from build123d import *

# Parameters (mm, degrees)
BOSS_EXTRUDE1_DEPTH       = 4.7625
F_8_32_TAPPED_HOLE1_D     = 3.4544
F_8_32_TAPPED_HOLE1_DEPTH = 8.89
F_8_32_TAPPED_HOLE1_TIP   = 1.037806461
BOSS_EXTRUDE2_DEPTH       = 9.525
SKETCH5_W                 = 6.4262
SKETCH5_H                 = 22.225
CUT_EXTRUDE1_DEPTH        = 6.223
CUT_EXTRUDE2_DEPTH        = 1.5875
CUT_EXTRUDE4_DEPTH        = 5.7625
CUT_EXTRUDE4_DEPTH_BACK   = 5.7625
FILLET1_R                 = 1.524
BOSS_EXTRUDE3_DEPTH       = 6.35
FILLET2_R                 = 0.254
CUT_EXTRUDE5_DEPTH        = 8.9375


with BuildPart() as part:
    # Sketch1 → Boss-Extrude1 (new body, symmetric)
    with BuildSketch(Plane(origin=(0, 0, 0), x_dir=(0, 0, -1), z_dir=(1, 0, 0))):
        with BuildLine():
            Line((-18.389854, 0), (18.389854, 0))
            Line((18.389854, 0), (18.389854, -18.35404))
            ThreePointArc((18.389854, -18.35404), (3.13664885, -20.715801882), (-11.682560966, -25.031958383))
            Line((-11.682560966, -25.031958383), (-18.389854, 0))
        make_face()
    extrude(amount=BOSS_EXTRUDE1_DEPTH, both=True)

    # #8-32 Tapped Hole1
    with Locations(Plane(origin=(0, 0, 0), x_dir=(-1, 0, 0), z_dir=(0, 1, 0))):
        with Locations((0, 12.090146)):
            Hole(F_8_32_TAPPED_HOLE1_D / 2, depth=F_8_32_TAPPED_HOLE1_DEPTH)
            with Locations((0, 0, -(F_8_32_TAPPED_HOLE1_DEPTH + F_8_32_TAPPED_HOLE1_TIP / 2))):  # 118° drill point
                Cone(0, F_8_32_TAPPED_HOLE1_D / 2, F_8_32_TAPPED_HOLE1_TIP, mode=Mode.SUBTRACT)

    # Sketch4 → Boss-Extrude2 (add)
    with BuildSketch(Plane(origin=(4.7625, 0, 0), x_dir=(0, 0, -1), z_dir=(1, 0, 0))):
        with BuildLine():
            Line((18.389854, 0), (24.739854, 0))
            Line((24.739854, 0), (24.739854, -17.95993887))
            ThreePointArc((24.739854, -17.95993887), (21.562219751, -18.114544788), (18.389854, -18.35404))
            Line((18.389854, -18.35404), (18.389854, 0))
        make_face()
    extrude(amount=-BOSS_EXTRUDE2_DEPTH)

    # Sketch5 → Cut-Extrude1 (cut)
    with BuildSketch(Plane(origin=(0, 0, -24.739854), x_dir=(-1, 0, 0), z_dir=(0, 0, -1))):
        with Locations((0, -11.1125)):
            Rectangle(SKETCH5_W, SKETCH5_H)
    extrude(amount=-CUT_EXTRUDE1_DEPTH, mode=Mode.SUBTRACT)

    # Sketch6 → Cut-Extrude2 (cut)
    with BuildSketch(Plane(origin=(4.7625, -3.455581552, 12.676714301), x_dir=(0, -0.262996683, 0.964796738), z_dir=(-1, 0, 0))):
        with BuildLine():
            Line((4.603212059, 4.836470596), (-1.739365308, 3.107529419))
            Line((-1.739365308, 3.107529419), (-1.636225637, -20.725696455))
            ThreePointArc((-1.636225637, -20.725696455), (1.5419234, -20.859537189), (4.715359636, -21.078277005))
            Line((4.715359636, -21.078277005), (4.603212059, 4.836470596))
        make_face()
    cut_extrude2 = extrude(amount=CUT_EXTRUDE2_DEPTH, mode=Mode.SUBTRACT)

    # Mirror1: Cut-Extrude2 across plane
    add(cut_extrude2.mirror(Plane(origin=(0, 0, 0), x_dir=(0, 0, 1), z_dir=(1, 0, 0))), mode=Mode.SUBTRACT)

    # Sketch8 → Cut-Extrude4 (cut, two sides)
    with BuildSketch(Plane(origin=(0, 0, 0), x_dir=(0, 0, -1), z_dir=(1, 0, 0))) as cut_extrude4_sk:
        with BuildLine():
            Line((-8.120493812, -1.524), (17.119854, -1.524))
            Line((17.119854, -1.524), (17.119854, -16.942404249))
            ThreePointArc((17.119854, -16.942404249), (6.985210432, -18.377350774), (-2.991129125, -20.667049623))
            Line((-2.991129125, -20.667049623), (-8.120493812, -1.524))
        make_face()
    extrude(amount=CUT_EXTRUDE4_DEPTH, mode=Mode.SUBTRACT)
    extrude(cut_extrude4_sk.sketch, amount=-CUT_EXTRUDE4_DEPTH_BACK, mode=Mode.SUBTRACT)

    # Fillet1
    fillet1_edges = [part.edges().sort_by_distance(p)[0] for p in [
        (0, -20.667049623, 2.991129125),
        (0, -1.524, 8.120493812),
        (0, -1.524, -17.119854),
        (0, -16.942404249, -17.119854),
    ]]
    fillet(fillet1_edges, radius=FILLET1_R)

    # Sketch9 → Boss-Extrude3 (add)
    with BuildSketch(Plane(origin=(3.175, 0, 0), x_dir=(0, 0, -1), z_dir=(1, 0, 0))):
        Polygon((-18.389854, 0), (-21.676855873, 0), (-21.095098292, -2.171148848), (-18.028283794, -1.349398379), align=None)
    extrude(amount=-BOSS_EXTRUDE3_DEPTH)

    # Fillet2
    fillet2_edges = [part.edges().sort_by_distance(p)[0] for p in [
        (0, -2.171148848, 21.095098292),
    ]]
    fillet(fillet2_edges, radius=FILLET2_R)

    # Sketch13 → Cut-Extrude5 (cut, through all)
    with BuildSketch(Plane(origin=(3.175, 0, 0), x_dir=(0, 0, -1), z_dir=(1, 0, 0))):
        with BuildLine():
            Line((-17.905611214, -1.316528361), (-18.028283794, -1.349398379))
            Line((-18.028283794, -1.349398379), (-11.682560966, -25.031958383))
            ThreePointArc((-11.682560966, -25.031958383), (-11.622647023, -25.010220768), (-11.562721445, -24.988515246))
            Line((-11.562721445, -24.988515246), (-17.905611214, -1.316528361))
        make_face()
    extrude(amount=-CUT_EXTRUDE5_DEPTH, mode=Mode.SUBTRACT)


solid = part.part
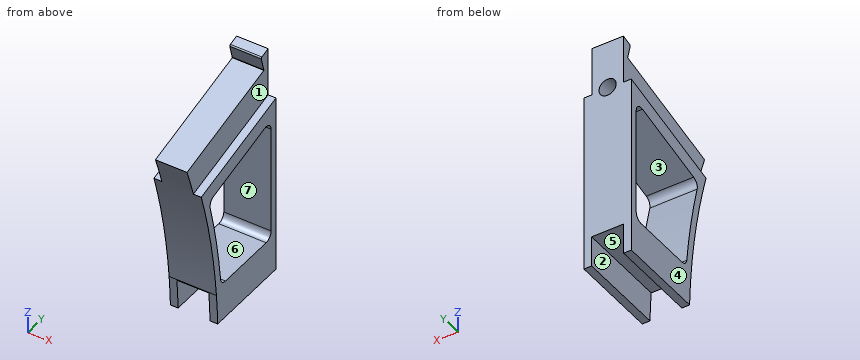
The listing builds one solid part. Answer for the finished solid, in the listing's coordinates (mm). Face numbers are marked on the shaded views. A direction names the side the tool comes from. Coordinates: 2 decimals unless noted, no trailing zeros. Write each loop counter-clockwise with the first axis right and the second up, starting at its lowest first coordinate (ties: lowest second). Pieces come first, ordered by that corner, then holes. Notation, with made-up numbers: (32.25, 27.25) - (57.25, 27.25) arc R14 cw to (57.25, 40.25) - close; hole circle Ø4 at (85, 22.25). An arc over 180 degrees is marked (long way). Put each result on its own line as item: value.
1. The part is cut by section D-D on y = -13.5. Give the vertices of the cut face in (x, z) (1 decimal), plus the area to 3 significant figures.
Answer sheet:
outline: (-4.8, -24.7) - (-3.2, -24.7) - (-3.2, -18.5) - (3.2, -18.5) - (3.2, -24.7) - (4.8, -24.7) - (4.8, -17.1) - (-4.8, -17.1) - close; (-4.8, 4.9) - (4.8, 4.9) - (4.8, 8.2) - (3.2, 8.2) - (3.2, 14.6) - (-3.2, 14.6) - (-3.2, 8.2) - (-4.8, 8.2) - close
area: 105 mm^2
2. The part is cut by section C-C on z = -2.5. Give the vertices of the cut face in (x, y), plus the area to 3 significant figures.
Answer sheet:
outline: (-4.76, -20.86) - (4.76, -20.86) - (4.76, -19.3) - (-4.76, -19.3) - close; (-4.76, -1.52) - (4.76, -1.52) - (4.76, 0) - (-4.76, 0) - close
area: 29.4 mm^2
3. Flat-ended cylindrical pins translate along their axes: pin 1 Ø2 at (x, z) = (0, 12.09) entering from -Y; pin 2 Ø8 at (y, z) = (-14.5, 13) entering from -X (3 decimals); pin 3 Ø5 at (x, y) = (0.5, -6.5) entering from +Z. Find the tip coordinate at first contact, or state that the pin passes through.
Answer sheet:
pin 1: stops at y = -24.99
pin 2: stops at x = -3.175
pin 3: stops at z = 17.19
4. The part is cut by section B-B on x = 4. Give the vertices of the cut face in (y, z) (1 decimal).
Answer sheet:
outline: (-23, 5.6) arc R119 cw to (-18.4, -18.4) arc R119 cw to (-18, -24.7) - (0, -24.7) - (0, 11.8) - close; hole (-20.3, 1.5) arc R120.5 cw to (-17.1, -15.8) arc R1.5 ccw to (-15.6, -17.1) - (-3, -17.1) arc R1.5 ccw to (-1.5, -15.6) - (-1.5, 6.1) arc R1.5 ccw to (-3.4, 7.6) - (-19.2, 3.4) arc R1.5 ccw to start
5. Determine the mould class of the marked faces 4, 5, 6 and 7 for opening direction Z: pulls with the +Z half, pulls with the -Z half, needs draft (parallel to the pull), parting line crosses it, or undercut.
Answer sheet:
face 4: needs draft
face 5: pulls with the -Z half
face 6: undercut
face 7: undercut
6. The part is cut by section A-A on y = -6.25. Give the vertices of the cut face in (x, z) (1 decimal), plus the area to 3 significant figures.
Answer sheet:
outline: (-4.8, -24.7) - (-3.2, -24.7) - (-3.2, -18.5) - (3.2, -18.5) - (3.2, -24.7) - (4.8, -24.7) - (4.8, -17.1) - (-4.8, -17.1) - close; (-4.8, 6.9) - (4.8, 6.9) - (4.8, 10.1) - (3.2, 10.1) - (3.2, 16.6) - (-3.2, 16.6) - (-3.2, 10.1) - (-4.8, 10.1) - close; hole circle Ø3.5 at (0, 12.1)
area: 95.4 mm^2
7. Find the intervals of material crossed by line 1 along Z through (x, y) = (0, -7); line 2 along Z through (x, y) = (0, -2.5); line 3 along X through (y, z) = (-10.75, 11) (3 decimals), in increasing order. Write a range as from..to.
Answer sheet:
line 1: z = -18.52..-17.12, 6.65..10.36, 13.82..16.38
line 2: z = -18.52..-17.02, 7.56..10.36, 13.82..17.59
line 3: x = -3.175..3.175
8. A tool of negligible diameter and unlimited length cuts with its end or side. For the marked faces 1, 2 and 3, from which of +Z, -Z, +X, -X, +Y, -Y can it reach the whole face along a straight path? Write none if from no direction.
Answer sheet:
face 1: +Z, +X, -Y
face 2: -Z, +Y, -Y
face 3: +X, -X
